from build123d import *

# Parameters (mm, degrees)
CROQUIS1_W              = 51
CROQUIS1_H              = 5
SALIENTE_EXTRUIR1_DEPTH = 4.4
CROQUIS2_R              = 0.57
CORTAR_EXTRUIR1_DEPTH   = 26.997307553


with BuildPart() as part:
    # Croquis1 → Saliente-Extruir1 (new body)
    with BuildSketch(Plane.XY):
        Rectangle(CROQUIS1_W, CROQUIS1_H)
    extrude(amount=SALIENTE_EXTRUIR1_DEPTH)

    # Croquis2 → Cortar-Extruir1 (cut, through all)
    with BuildSketch(Plane.XY.offset(4.4)):
        with Locations((-24.13, 1.27)):
            Circle(CROQUIS2_R)
        with Locations((-21.59, 1.27)):
            Circle(CROQUIS2_R)
        with Locations((-19.05, 1.27)):
            Circle(CROQUIS2_R)
        with Locations((-16.51, 1.27)):
            Circle(CROQUIS2_R)
        with Locations((-13.97, 1.27)):
            Circle(CROQUIS2_R)
        with Locations((-11.43, 1.27)):
            Circle(CROQUIS2_R)
        with Locations((-8.89, 1.27)):
            Circle(CROQUIS2_R)
        with Locations((-6.35, 1.27)):
            Circle(CROQUIS2_R)
        with Locations((-3.81, 1.27)):
            Circle(CROQUIS2_R)
        with Locations((-1.27, 1.27)):
            Circle(CROQUIS2_R)
        with Locations((1.27, 1.27)):
            Circle(CROQUIS2_R)
        with Locations((3.81, 1.27)):
            Circle(CROQUIS2_R)
        with Locations((6.35, 1.27)):
            Circle(CROQUIS2_R)
        with Locations((8.89, 1.27)):
            Circle(CROQUIS2_R)
        with Locations((11.43, 1.27)):
            Circle(CROQUIS2_R)
        with Locations((13.97, 1.27)):
            Circle(CROQUIS2_R)
        with Locations((16.51, 1.27)):
            Circle(CROQUIS2_R)
        with Locations((19.05, 1.27)):
            Circle(CROQUIS2_R)
        with Locations((21.59, 1.27)):
            Circle(CROQUIS2_R)
        with Locations((24.13, 1.27)):
            Circle(CROQUIS2_R)
        with Locations((-21.59, -1.27)):
            Circle(CROQUIS2_R)
        with Locations((-19.05, -1.27)):
            Circle(CROQUIS2_R)
        with Locations((-16.51, -1.27)):
            Circle(CROQUIS2_R)
        with Locations((-13.97, -1.27)):
            Circle(CROQUIS2_R)
        with Locations((-11.43, -1.27)):
            Circle(CROQUIS2_R)
        with Locations((-8.89, -1.27)):
            Circle(CROQUIS2_R)
        with Locations((-6.35, -1.27)):
            Circle(CROQUIS2_R)
        with Locations((-3.81, -1.27)):
            Circle(CROQUIS2_R)
        with Locations((-1.27, -1.27)):
            Circle(CROQUIS2_R)
        with Locations((1.27, -1.27)):
            Circle(CROQUIS2_R)
        with Locations((3.81, -1.27)):
            Circle(CROQUIS2_R)
        with Locations((6.35, -1.27)):
            Circle(CROQUIS2_R)
        with Locations((8.89, -1.27)):
            Circle(CROQUIS2_R)
        with Locations((11.43, -1.27)):
            Circle(CROQUIS2_R)
        with Locations((13.97, -1.27)):
            Circle(CROQUIS2_R)
        with Locations((16.51, -1.27)):
            Circle(CROQUIS2_R)
        with Locations((19.05, -1.27)):
            Circle(CROQUIS2_R)
        with Locations((21.59, -1.27)):
            Circle(CROQUIS2_R)
        with Locations((24.13, -1.27)):
            Circle(CROQUIS2_R)
        with Locations((-24.13, -1.27)):
            Circle(CROQUIS2_R)
    extrude(amount=-CORTAR_EXTRUIR1_DEPTH, mode=Mode.SUBTRACT)


solid = part.part
Input: part model. Units: mm. Frame: model coordinates. Coordinates: 2 decimals unless noted, no trailing zeros. Order: outer loops, then holes, each group sorted by start corner. A loop starts at its lowest first (then second) coordinate and runs counter-clockwise, first axis right, second up. Notation, with made-up numbers: M -32.5,27.25 L -28.5,27.25 A24 cw -28.5,55.25 Z; hole C 55.5,-27 d7. An arc over 180 degrees is marked long. One line per question, with ' | ' between items.
Item 1: Section A-A (x = 24.13). Output: boundary loops of the cut face in (y, z), then the cut area to 3 significant figures.
Geometry results:
outline: M -2.5,0 L -1.84,0 L -1.84,4.4 L -2.5,4.4 Z; M -0.7,0 L 0.7,0 L 0.7,4.4 L -0.7,4.4 Z; M 1.84,0 L 2.5,0 L 2.5,4.4 L 1.84,4.4 Z | area: 12.0 mm^2
Item 2: Section B-B (y = -1.27). Give the number of separate pieces and of enclosed holes in the cut face, then the cut area to 3 significant figures.
Geometry results:
separate pieces: 21 | enclosed holes: 0 | area: 124 mm^2
Item 3: Pin query (flat end, axial travel): pin 1 (1.3 mm diameter, centred on x = -24.13, y = 1.27, fed in from +Z). Return the tip coordinate at first contact, or that it passes through.
Geometry results:
pin 1: stops at z = 4.4
Item 4: Draft query along Y for faces 1 (the cylindrical face through (0.85, 1.655, 2.231)), 2 (the flat face through (0, 2.5, 2)), 3 (the cylindrical face through (11.356, 1.835, 2.231)), 4 (the flat face through (25.5, 0, 2)). Return one class per face: released by +Y, released by -Y, zero draft, split by the parting line, or undercut.
Geometry results:
face 1: undercut | face 2: released by +Y | face 3: undercut | face 4: zero draft
Item 5: Ray query, line 1 along Y through (x, z) = (21.59, 1.8). Return the intervals inside material, ascending.
Geometry results:
line 1: y = -2.5 to -1.84, -0.7 to 0.7, 1.84 to 2.5
